from build123d import *

# Parameters (mm, degrees)
SKETCH1_W           = 14.5
SKETCH1_H           = 10
BOSS_EXTRUDE1_DEPTH = 2.5
SKETCH2_R           = 1.9
CUT_EXTRUDE1_DEPTH  = 10.154916712
SKETCH3_W           = 2
SKETCH3_H           = 10
BOSS_EXTRUDE2_DEPTH = 2.5
FILLET1_R           = 2
FILLET2_R           = 2


with BuildPart() as part:
    # Sketch1 → Boss-Extrude1 (new body)
    with BuildSketch(Plane(origin=(0, 0, 0), x_dir=(1, 0, 0), z_dir=(0, 1, 0))):
        Rectangle(SKETCH1_W, SKETCH1_H)
    extrude(amount=BOSS_EXTRUDE1_DEPTH)

    # Sketch2 → Cut-Extrude1 (cut, through all)
    with BuildSketch(Plane(origin=(0, 2.5, 0), x_dir=(1, 0, 0), z_dir=(0, 1, 0))):
        with Locations(Location((2.323455921, 0, 0), (0, 0, 270))):
            Circle(SKETCH2_R)
    extrude(amount=-CUT_EXTRUDE1_DEPTH, mode=Mode.SUBTRACT)

    # Sketch3 → Boss-Extrude2 (add)
    with BuildSketch(Plane(origin=(0, 2.5, 0), x_dir=(1, 0, 0), z_dir=(0, 1, 0))):
        with Locations((-6.25, 0)):
            Rectangle(SKETCH3_W, SKETCH3_H)
    extrude(amount=BOSS_EXTRUDE2_DEPTH)

    # Fillet1
    fillet1_edges = [part.edges().sort_by_distance(p)[0] for p in [
        (-5.25, 2.5, 0),
    ]]
    fillet(fillet1_edges, radius=FILLET1_R)

    # Fillet2
    fillet2_edges = [part.edges().sort_by_distance(p)[0] for p in [
        (7.25, 1.25, 5),
        (7.25, 1.25, -5),
    ]]
    fillet(fillet2_edges, radius=FILLET2_R)


solid = part.part
Read the model definition and answer for the solid it produces. Units are mm, in the model's axes. A direction names the side the tool comes from. Coordinates: 2 decimals unless noted, no trailing zeros. Write each loop counter-clockwise with the first axis right and the second up, starting at its lowest first coordinate (ties: lowest second). Pieces come first, ordered by that corner, then holes. Notation, with made-up numbers: (53, 75) - (99, 75) arc R25 cw to (99, 110) - close; hole circle Ø4 at (45, 64.5). An arc over 180 degrees is marked (long way). One line per question, with ' | ' between items.
Q1. Find section B-B, the plane x = 3.25. Write down the section's boundary in (y, z).
Result set:
outline: (0, -5) - (2.5, -5) - (2.5, -1.66) - (0, -1.66) - close; (0, 1.66) - (2.5, 1.66) - (2.5, 5) - (0, 5) - close
Q2. For faces 5 (the flat face through (1.9, 2.5, 2.2)), 6 (the flat face through (0, 0, 0)), determine the directions among +Z, -Z, +X, -X, +Y, -Y from which every point of the face is accessible in a straight line to the end or side of a thin tool.
Result set:
face 5: +Z, -Z, +X, +Y | face 6: +Z, -Z, +X, -X, -Y
Q3. Determine the mould class of faces 1 (the cylindrical face through (6.68, 1.27, -4.4)), 2 (the cylindrical face through (6.65, 1.27, 4.43)), 3 (the flat face through (7.25, 1, 0)), 4 (the cylindrical face through (4.207, 1.268, -0.247)) for opening direction Z: +Z half, -Z half, draft (parallel to the pull), parting line (faces both ways), or undercut.
Result set:
face 1: -Z half | face 2: +Z half | face 3: draft | face 4: undercut
Q4. Each of these flat-tipped pins is pushed along its axis until it touches: P1, Ø3, axis at x = -0.5, z = -2, coming from the +Y side; P2, Ø3.5, axis at x = 2.32, z = 0, coming from the -Y side. Where does it stop, or does it pass through?
Result set:
P1: y = 2.5 | P2: through
Q5. Find section C-C, the plane z = 2.5. Write down the section's boundary in (x, y).
Result set:
outline: (-7.25, 0) - (7.25, 0) - (7.25, 2.5) - (-3.25, 2.5) arc R2 cw to (-5.25, 4.5) - (-5.25, 5) - (-7.25, 5) - close
Q6. Find section D-D, the plane y = 0.9. Write down the section's boundary in (x, z).
Result set:
outline: (-7.25, -5) - (5.25, -5) arc R2 ccw to (7.25, -3) - (7.25, 3) arc R2 ccw to (5.25, 5) - (-7.25, 5) - close; hole circle Ø3.8 at (2.32, 0)
Q7. Consider L1, parallel to X at y = 1.35, z = 0; L2, parallel to Y at x = 3.25, z = -2.75; L3, parallel to X at y = 1.15, z = -1. Determine where each line is inside the solid, lowest interval first. Write a range as [from, to].
Result set:
L1: [-7.25, 0.42], [4.22, 7.25] | L2: [0, 2.5] | L3: [-7.25, 0.71], [3.94, 7.25]
Q8. Find section A-A, the plane z = 0. Write down the section's boundary in (x, y), plus the area to 3 significant figures.
Result set:
outline: (-7.25, 0) - (0.42, 0) - (0.42, 2.5) - (-3.25, 2.5) arc R2 cw to (-5.25, 4.5) - (-5.25, 5) - (-7.25, 5) - close; (4.22, 0) - (7.25, 0) - (7.25, 2.5) - (4.22, 2.5) - close | area: 32.6 mm^2
